```python
from build123d import *

# Parameters (mm, degrees)
SKETCH1_W               = 180
SKETCH1_H               = 10
BOSS_EXTRUDE1_DEPTH     = 15
SKETCH2_W               = 17
SKETCH2_H               = 15
CUT_EXTRUDE1_DEPTH      = 3
SKETCH3_W               = 3
SKETCH3_H               = 10
BOSS_EXTRUDE2_DEPTH     = 5.5
SKETCH4_W               = 6
SKETCH4_H               = 3.5
CUT_EXTRUDE2_DEPTH      = 7
LPATTERN1_COUNT         = 4
LPATTERN1_PITCH         = 30
MIRROR1_COPY_1_SKETCH_W = 3
MIRROR1_COPY_1_SKETCH_H = 10
MIRROR1_COPY_1_DEPTH    = 5.5
MIRROR1_COPY_2_SKETCH_W = 3
MIRROR1_COPY_2_SKETCH_H = 10
MIRROR1_COPY_2_DEPTH    = 5.5
MIRROR1_COPY_3_SKETCH_W = 3
MIRROR1_COPY_3_SKETCH_H = 10
MIRROR1_COPY_3_DEPTH    = 5.5
MIRROR1_COPY_4_SKETCH_W = 6
MIRROR1_COPY_4_SKETCH_H = 3.5
MIRROR1_COPY_4_DEPTH    = 7
MIRROR1_COPY_5_SKETCH_W = 6
MIRROR1_COPY_5_SKETCH_H = 3.5
MIRROR1_COPY_5_DEPTH    = 7
MIRROR1_COPY_6_SKETCH_W = 6
MIRROR1_COPY_6_SKETCH_H = 3.5
MIRROR1_COPY_6_DEPTH    = 7


with BuildPart() as part:
    # Sketch1 → Boss-Extrude1 (new body)
    with BuildSketch(Plane(origin=(0, 0, 0), x_dir=(1, 0, 0), z_dir=(0, 1, 0))):
        Rectangle(SKETCH1_W, SKETCH1_H)
    extrude(amount=BOSS_EXTRUDE1_DEPTH)

    # Sketch2 → Cut-Extrude1 (cut)
    with BuildSketch(Plane(origin=(0, 0, -5), x_dir=(-1, 0, 0), z_dir=(0, 0, -1))):
        with Locations((-81.5, 7.5)):
            Rectangle(SKETCH2_W, SKETCH2_H)
    extrude(amount=-CUT_EXTRUDE1_DEPTH, mode=Mode.SUBTRACT)

    # Sketch3 → Boss-Extrude2 (add)
    with BuildSketch(Plane(origin=(0, 15, 0), x_dir=(1, 0, 0), z_dir=(0, 1, 0))):
        with Locations((44.673610622, 0)):
            Rectangle(SKETCH3_W, SKETCH3_H)
    boss_extrude2 = extrude(amount=BOSS_EXTRUDE2_DEPTH)

    # Sketch4 → Cut-Extrude2 (cut)
    with BuildSketch(Plane(origin=(46.173610622, 0, 0), x_dir=(0, 0, -1), z_dir=(1, 0, 0))):
        with Locations((0, 16.75)):
            Rectangle(SKETCH4_W, SKETCH4_H)
    cut_extrude2 = extrude(amount=-CUT_EXTRUDE2_DEPTH, mode=Mode.SUBTRACT)

    # LPattern1: Boss-Extrude2, Cut-Extrude2 ×4
    with Locations(*[(-i * LPATTERN1_PITCH, 0, 0) for i in range(1, LPATTERN1_COUNT)]):
        add(boss_extrude2)
        add(cut_extrude2, mode=Mode.SUBTRACT)

    # Mirror1: Boss-Extrude2, Cut-Extrude2 across plane
    add(boss_extrude2.mirror(Plane(origin=(0, 7.5, 0), x_dir=(0, 0, 1), z_dir=(0, -1, 0))))
    add(cut_extrude2.mirror(Plane(origin=(0, 7.5, 0), x_dir=(0, 0, 1), z_dir=(0, -1, 0))), mode=Mode.SUBTRACT)

    # Mirror1 copy 1 sketch → Mirror1 copy 1 (add)
    with BuildSketch(Plane(origin=(-30, 0, 0), x_dir=(1, 0, 0), z_dir=(0, -1, 0))):
        with Locations((44.673610622, 0)):
            Rectangle(MIRROR1_COPY_1_SKETCH_W, MIRROR1_COPY_1_SKETCH_H)
    extrude(amount=MIRROR1_COPY_1_DEPTH)

    # Mirror1 copy 2 sketch → Mirror1 copy 2 (add)
    with BuildSketch(Plane(origin=(-60, 0, 0), x_dir=(1, 0, 0), z_dir=(0, -1, 0))):
        with Locations((44.673610622, 0)):
            Rectangle(MIRROR1_COPY_2_SKETCH_W, MIRROR1_COPY_2_SKETCH_H)
    extrude(amount=MIRROR1_COPY_2_DEPTH)

    # Mirror1 copy 3 sketch → Mirror1 copy 3 (add)
    with BuildSketch(Plane(origin=(-90, 0, 0), x_dir=(1, 0, 0), z_dir=(0, -1, 0))):
        with Locations((44.673610622, 0)):
            Rectangle(MIRROR1_COPY_3_SKETCH_W, MIRROR1_COPY_3_SKETCH_H)
    extrude(amount=MIRROR1_COPY_3_DEPTH)

    # Mirror1 copy 4 sketch → Mirror1 copy 4 (cut)
    with BuildSketch(Plane(origin=(16.173610622, 15, 0), x_dir=(0, 0, -1), z_dir=(1, 0, 0))):
        with Locations((0, -16.75)):
            Rectangle(MIRROR1_COPY_4_SKETCH_W, MIRROR1_COPY_4_SKETCH_H)
    extrude(amount=-MIRROR1_COPY_4_DEPTH, mode=Mode.SUBTRACT)

    # Mirror1 copy 5 sketch → Mirror1 copy 5 (cut)
    with BuildSketch(Plane(origin=(-13.826389378, 15, 0), x_dir=(0, 0, -1), z_dir=(1, 0, 0))):
        with Locations((0, -16.75)):
            Rectangle(MIRROR1_COPY_5_SKETCH_W, MIRROR1_COPY_5_SKETCH_H)
    extrude(amount=-MIRROR1_COPY_5_DEPTH, mode=Mode.SUBTRACT)

    # Mirror1 copy 6 sketch → Mirror1 copy 6 (cut)
    with BuildSketch(Plane(origin=(-43.826389378, 15, 0), x_dir=(0, 0, -1), z_dir=(1, 0, 0))):
        with Locations((0, -16.75)):
            Rectangle(MIRROR1_COPY_6_SKETCH_W, MIRROR1_COPY_6_SKETCH_H)
    extrude(amount=-MIRROR1_COPY_6_DEPTH, mode=Mode.SUBTRACT)


solid = part.part
```
Could you check a few things on this model? Use its own coordinates, in mm. A direction names the side the tool comes from. Round coordinates to 2 decimals unless told otherwise and drop trailing zeros. Order: outer loops, then holes, each group sorted by start corner. A loop starts at its lowest first (then second) coordinate and runs counter-clockwise, first axis right, second up. Notation, with made-up numbers: (-14, 42.25) -> (-9, 42.25) arc R19 ccw to (-9, 55.25) -> close; hole circle Ø6 at (88, 81). An arc over 180 degrees is marked (long way). One line per question, with ' | ' between items.
Q1. If I drill on line 1 (X direction, y = -0.5, z = -3.25); line 2 (Y direction, x = -44.5, z = -1); line 3 (Y direction, x = 59, z = -1.25), over which ranges is the centre line in solid material (lowest first)? Write a range as from..to.
Computed values:
line 1: -46.83..-43.83, -16.83..-13.83, 13.17..16.17, 43.17..46.17 | line 2: -5.5..-3.5, 0..15, 18.5..20.5 | line 3: 0..15
Q2. I'm going to push flat-ended pins straight in: pin 1 (0.9 mm diameter, centred on y = 11, z = -3, fed in from +X); pin 2 (1.6 mm diameter, centred on y = 18, z = -0.5, fed in from -X); pin 3 (5 mm diameter, centred on x = 38.5, z = -2.5, fed in from +Y). Where does each tip first touch, or does it pass through?
Computed values:
pin 1: x = 73 | pin 2: x = -46.83 | pin 3: y = 15
Q3. We'd pull the mould along Y, two halves only. Please class faces 6 (the face through (-45, -5.5, 0)), 7 (the face through (-10, 7, -5)), 8 (the face through (45, 17, 3)): released by +Y, released by -Y, zero draft, split by the parting line, or undercut.
Computed values:
face 6: released by -Y | face 7: zero draft | face 8: undercut
Q4. If we section it at A-A on z = -0.25: Give the number of separate pieces and of enclosed holes in the cut face, plus the area to 3 significant figures.
Computed values:
separate pieces: 9 | enclosed holes: 0 | area: 2,750 mm²
Q5. Which directions (+Z, -Z, +X, -X, +Y, -Y) give clear straight access to the entire face, cutting with the end or side of a thin tool? Please do faces 1 (the face through (46.174, 19, 0)), 2 (the face through (13.174, 19, 0)), 3 (the face through (43.174, -4, 0)), 4 (the face through (82, 8, -2)), 5 (the face through (45, -3.5, 0)).
Computed values:
face 1: +Z, -Z, +X, +Y | face 2: +Z, -Z, +Y | face 3: +Z, -Z, -Y | face 4: -Z, +X, +Y, -Y | face 5: +X, -X
Q6. If we section it at B-B on y = 1.5: Write out the boundary of the cut face in (x, z), plus the area to 3 significant figures.
Computed values:
outline: (-90, -5) -> (73, -5) -> (73, -2) -> (90, -2) -> (90, 5) -> (-90, 5) -> close | area: 1,750 mm²
Q7. If we section it at C-C on x = 58: Write out the boundary of the cut face in (y, z).
Computed values:
outline: (0, -5) -> (15, -5) -> (15, 5) -> (0, 5) -> close
